The figure shows three views and two pictorial views of one solid part (mm, origin at its lowest corner). Answer the questions. A direction names the side the tool comes from. Coordinates: 2 decimals unless noted, no trailing zeros. Write each loop counter-clockwise with the first axis right and the second up, starting at its lowest first coordinate (ties: lowest second). Pieces come first, ordered by that corner, then holes.
Item 1: Section C-C (z = 20.5) is taken. Give the vertices of the cut face in (x, y), then the cut area to 3 significant figures.
Item 2: A tool of negligible diameter and unlimited length cuts with its end or side. For the marked faces 1, 2 and 3, from which of +Z, -Z, +X, -X, +Y, -Y can it reach the whole face along a straight path? Write none if from no direction.
Item 3: Straight lines are drawn through the part: probe 1 along Z at (x, y) = (64.5, 6.5); probe 2 along X at (y, z) = (2.5, 4.5); probe 3 along Z at (x, y) = (15, 5). For each, find the intervals that lie inside material, in ascending order.
Item 4: Determine the mould class of the marked faces 4, 5 and 6 for opening direction Y: released by +Y, released by -Y, zero draft, split by the parting line, or undercut.
Item 5: Each of these flat-tipped pins is pushed along its axis until it touches: P1, Ø2, axis at y = 5, z = 20, coming from the -X side; P2, Ø2.5, axis at x = 64.5, z = 20.5, coming from the -Y side; P3, Ø4, axis at x = 56, y = 3.5, coming from the +Z side. Where does it stop, or does it pass through?
Item 6: Section A-A (x = 64.5) is taken. Give the vertices of the cut face in (y, z), then the cut area to 3 significant figures.
Item 7: Section B-B (y = 3.5) is taken. Give the vertices of the cut face in (x, z) (3 decimals).
Item 8: Section D-D (z = 15) is taken. Give the vertices of the cut face in (x, y) (3 decimals), then the cut area to 3 significant figures.
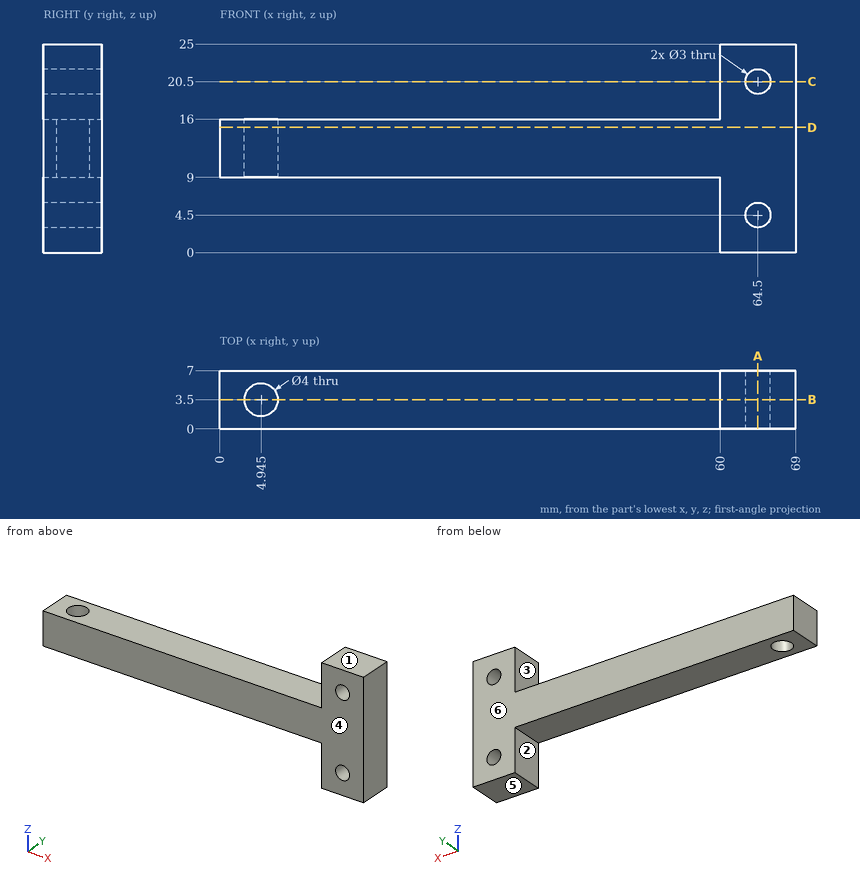
Established:
1. outline: (60, 0) - (63, 0) - (63, 7) - (60, 7) - close; (66, 0) - (69, 0) - (69, 7) - (66, 7) - close
1. area: 42.0 mm2
2. face 1: +Z, +X, -X, +Y, -Y
2. face 2: -Z, -X, +Y, -Y
2. face 3: +Z, -X, +Y, -Y
3. probe 1: z = 0 to 3, 6 to 19, 22 to 25
3. probe 2: x = 60 to 63, 66 to 69
3. probe 3: z = 9 to 16
4. face 4: released by -Y
4. face 5: zero draft
4. face 6: released by +Y
5. P1: stops at x = 60
5. P2: passes through
5. P3: stops at z = 16
6. outline: (0, 0) - (7, 0) - (7, 3) - (0, 3) - close; (0, 6) - (7, 6) - (7, 19) - (0, 19) - close; (0, 22) - (7, 22) - (7, 25) - (0, 25) - close
6. area: 133 mm2
7. outline: (0, 9) - (2.945, 9) - (2.945, 16) - (0, 16) - close; (6.945, 9) - (60, 9) - (60, 0) - (69, 0) - (69, 25) - (60, 25) - (60, 16) - (6.945, 16) - close; hole circle Ø3 at (64.5, 4.5); hole circle Ø3 at (64.5, 20.5)
8. outline: (0, 0) - (69, 0) - (69, 7) - (0, 7) - close; hole circle Ø4 at (4.945, 3.5)
8. area: 470 mm2
